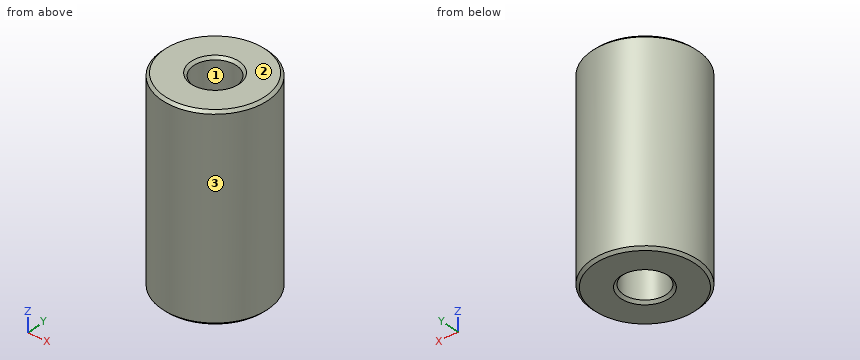
Autodesk Inventor part; units mm, degrees
ref_plane "YZ Plane" through (0, 0, 0) normal (1, 0, 0) x (0, 1, 0)
ref_plane "XZ Plane" through (0, 0, 0) normal (0, 1, 0) x (-1, 0, 0)
ref_plane "XY Plane" through (0, 0, 0) normal (0, 0, 1) x (1, 0, 0)
sketch "スケッチ1" plane through (0, 0, 0) normal (0, 0, 1) x (1, 0, 0)
  circle A0 centre (0, 0) radius 4
  dimension "d13" = 8
extrude "押し出し1" add sketch "スケッチ1" along normal blind 15
sketch "スケッチ2" plane through (0, 0, 15) normal (0, 0, 1) x (1, 0, 0)
  point P0 (0, 0)
  point P1 (0, 0)
hole "穴1" at (0, 0, 15) direction (0, 0, -1) diameter 3.242 end through all
chamfer "面取り1" distance 0.2 angle 45 4 edges at (0, 1.621, 15) (0, 1.621, 0) (-4, 0, 15) (-4, 0, 0)
properties part number "ARF-415" material "鋼、炭素鋼"
Check sheet for the modelled part. Datum: model origin and axes. Units: mm. Face numbers are marked on the shaded views. Coordinates: 2 decimals unless noted, no trailing zeros. Write each loop counter-clockwise with the first axis right and the second up, starting at its lowest first coordinate (ties: lowest second). Pieces come first, ordered by that corner, then holes. Notation, with made-up numbers: (-18.5, -22.5) -> (32.5, -22.5) arc R31 ccw to (32.5, 11.5) -> close; hole circle Ø4 at (30, -8.5). An arc over 180 degrees is marked (long way). Use a Markdown table: item, result.
1. Sectioned sample at A-A (y = 0). Enter the section's corners in (x, z).
Reported:
| item | result |
|---|---|
| outline | (-4, 0.2) -> (-3.8, 0) -> (-1.82, 0) -> (-1.62, 0.2) -> (-1.62, 14.8) -> (-1.82, 15) -> (-3.8, 15) -> (-4, 14.8) -> close; (1.62, 0.2) -> (1.82, 0) -> (3.8, 0) -> (4, 0.2) -> (4, 14.8) -> (3.8, 15) -> (1.82, 15) -> (1.62, 14.8) -> close |
2. Sectioned sample at C-C (z = 10.5). Enter the section's corners in (x, y), plus the area to 3 significant figures.
Reported:
| item | result |
|---|---|
| outline | circle Ø8 at (0, 0); hole circle Ø3.24 at (0, 0) |
| area | 42.0 mm2 |
3. Go/stop test with flat-tipped pins: pin 1 Ø2 at (x, y) = (1.5, 1.5) entering from -Z; pin 2 Ø1.5 at (x, z) = (2, 9.5) entering from -Y; pin 3 Ø1 at (y, z) = (-1.5, 3.5) entering from +X; pin 4 Ø2 at (y, z) = (1.5, 6) entering from +X. Record where each tip stops, or that it passes through.
Reported:
| item | result |
|---|---|
| pin 1 | stops at z = 0 |
| pin 2 | stops at y = -3.8 |
| pin 3 | stops at x = 3.87 |
| pin 4 | stops at x = 3.97 |
4. Release check for a two-part mould opening along Y. For the marked faces 1, 2 and 3 record: pulls with the +Y half, pulls with the -Y half, needs draft (parallel to the pull), parting line crosses it, or undercut.
Reported:
| item | result |
|---|---|
| face 1 | undercut |
| face 2 | needs draft |
| face 3 | parting line crosses it |
5. Scan lines: line 1 along Y through (x, z) = (0, 9.5); line 2 along X through (y, z) = (-1, 10.5); line 3 along Y through (x, z) = (-0.75, 1.5). Record each from-to range of solid material in increasing order.
Reported:
| item | result |
|---|---|
| line 1 | y = -4 to -1.62, 1.62 to 4 |
| line 2 | x = -3.87 to -1.28, 1.28 to 3.87 |
| line 3 | y = -3.93 to -1.44, 1.44 to 3.93 |
